Autodesk Inventor part; units mm, degrees
ref_plane "YZ Plane" through (0, 0, 0) normal (1, 0, 0) x (0, 1, 0)
ref_plane "XZ Plane" through (0, 0, 0) normal (0, 1, 0) x (-1, 0, 0)
ref_plane "XY Plane" through (0, 0, 0) normal (0, 0, 1) x (1, 0, 0)
sketch "Sketch1" plane through (0, 0, 0) normal (0, 0, 1) x (1, 0, 0)
  line L0 (0, 25.4) -> (-28.702, 25.4) construction
  line L1 (0, 25.4) -> (-86.36, 25.4) construction
  line L2 (-86.36, 25.4) -> (-80.01, 25.4) construction
  line L3 (-80.01, 25.4) -> (-73.66, 22.4389) construction
  line L4 (-80.01, 25.4) -> (-80.01, 22.4389) construction
  line L5 (-80.01, 0) -> (-86.36, 0)
  line L6 (-28.702, 59.6457) -> (-28.702, -91.9304) construction
  arc A0 (-28.9184, -4.2142) -> (-32.3684, 3.1843) centre (-35.052, -2.5707) ccw
  line L7 (-67.31, -147.4937) -> (-28.9184, -4.2142)
  line L8 (-80.01, 22.4389) -> (-73.66, 22.4389)
  line L9 (-80.01, 22.4389) -> (-80.01, 0)
  line L10 (-73.66, 22.4389) -> (-32.3684, 3.1843)
  line L11 (-28.702, -2.5707) -> (-60.452, -2.5707) construction
  line L12 (-60.452, 16.28) -> (-60.452, -121.8993) construction
  line L13 (-60.452, -121.8993) -> (-54.102, -121.8993) construction
  line L14 (-54.102, -121.8993) -> (-54.102, -98.2008) construction
  line L15 (-54.102, -98.2008) -> (-60.452, -98.2008)
  line L16 (-60.452, 16.28) -> (-60.452, 6.755) construction
  line L17 (-60.452, 16.28) -> (-60.452, 9.93) construction
  line L18 (-60.452, 9.93) -> (-46.8344, 9.93)
  line L19 (-60.452, 9.93) -> (-60.452, -98.2008)
  line L20 (-86.36, 0) -> (-86.36, -12.7) construction
  line L21 (-60.452, -12.7) -> (-73.152, -12.7) construction
  line L22 (-86.36, -12.7) -> (-86.36, -25.4) construction
  line L23 (-86.36, -25.4) -> (-86.36, -88.9) construction
  line L24 (-86.36, -88.9) -> (-73.66, -88.9) construction
  line L25 (-73.66, -88.9) -> (-73.66, -25.4) construction
  line L26 (-86.36, -25.4) -> (-73.66, -25.4)
  line L27 (-73.66, -25.4) -> (-73.66, -88.9)
  line L28 (-73.66, -88.9) -> (-86.36, -88.9)
  line L29 (-86.36, -12.7) -> (-73.152, -12.7)
  line L30 (-73.152, -133.7486) -> (-63.627, -133.7486)
  line L31 (-73.66, -88.9) -> (-73.66, -147.4937)
  line L32 (-73.66, -147.4937) -> (-67.31, -147.4937)
  line L33 (-73.152, -12.7) -> (-73.152, -133.7486)
  line L34 (-80.01, -25.4) -> (-80.01, -31.3436)
  line L35 (-80.01, -31.3436) -> (-86.36, -31.3436)
  line L36 (-86.36, 0) -> (-86.36, -25.4)
  line L37 (-86.36, -31.3436) -> (-86.36, -88.9)
  line L38 (0, -319.0244) -> (0, 122.7573)
  point P0 (0, 0)
  point P1 (-86.36, -255.9127)
  point P2 (-76.835, 22.4389)
  dimension "d0" = 28.702
  dimension "d1" = 86.36
  dimension "d2" = 6.35
  dimension "d3" = 25
  dimension "d5" = 25.4
  dimension "d6" = 25.4
  dimension "d8" = 12.7
  dimension "d11" = 6.35
  dimension "d12" = 31.75
  dimension "d13" = 6.35
  dimension "d15" = 6.35
  dimension "d16" = 12.7
  dimension "d17" = 12.7
  dimension "d18" = 12.7
  dimension "d19" = 63.5
  dimension "d20" = 12.7
  dimension "d22" = 9.525
  dimension "d23" = 6.35
  dimension "d25" = 5.9436
  dimension "d26" = 15
  dimension "d30" = 67.31
revolve "Revolution3" add sketch "Sketch1" angle 360 about axis through (0, -10, 0) along (0, 1, 0) contours L29 L33 L30 L7 L32 L31 L27 L26 L36
properties part number "Carrier Master Sketch"
For this review, take the finished solid that the model builds, in its own axes (mm). A direction names the side the tool comes from. Give positions to 0.01 mm unless a question says otherwise; leave off trailing zeros. Loops run counter-clockwise (first coordinate to the right, second up) from the corner with the lowest first, then second, coordinate; pieces in that order, holes last. Notation, with made-up numbers: M 58.25,76 L 96.25,76 A23 ccw 96.25,112 Z; hole C 21.5,46.25 d11. An arc over 180 degrees is marked long. Put each result on its own line as item: value. Start each with the question number.
(1) Wall thickness on L1, parallel to Z at x = 0, y = -69; L2, parallel to X at y = -95.5, z = 46; L3, parallel to X at y = -94, z = 3: over which ranges is each line inside the solid? List them lowest first.
(2) Add section C-C, the plane y = -48.5. Write out the cut boundary in (x, z).
(3) Machinability: for faces 1 (the cylindrical face through (15.86, -74.07, 71.41)), 2 (the flat face through (-64, -25.4, 39)), 3 (the flat face through (-32, -147.494, -60)), which of the approach directions +Z, -Z, +X, -X, +Y, -Y give a long, thin tool a straight path to every point of the face, cutting with its end or side? Answer none if there is none.
(4) Add section A-A, the plane x = 0. Write out the cut boundary in (y, z), then the cut area to 3 significant figures.
(5) For pin 1 (8 mm diameter, centred on y = -131, z = -49, fed in from +X); pin 2 (6 mm diameter, centred on x = 16, y = -97.5, fed in from +Z); pin 3 (2 mm diameter, centred on y = -51.5, z = -24, fed in from -X), all flat-tipped, find the tip position at first contact; note any pin that passes through.
(6) Add section B-B, the plane z = 0. Write out the cut boundary in (x, y), then the cut area to 3 significant figures.
Result:
1. L1: z = -73.66 to -73.15, 73.15 to 73.66
1. L2: x = -57.53 to -56.88, 56.88 to 57.53
1. L3: x = -73.6 to -73.09, 73.09 to 73.6
2. outline: C 0,0 d147.32; hole C 0,0 d146.3
3. face 1: +Y
3. face 2: -Y
3. face 3: +Z, -Z, +X, -X, -Y
4. outline: M -147.49,-73.66 L -25.4,-73.66 L -25.4,-86.36 L -12.7,-86.36 L -12.7,-73.15 L -133.75,-73.15 L -133.75,-63.63 L -147.49,-67.31 Z; M -147.49,67.31 L -133.75,63.63 L -133.75,73.15 L -12.7,73.15 L -12.7,86.36 L -25.4,86.36 L -25.4,73.66 L -147.49,73.66 Z
4. area: 671 mm^2
5. pin 1: stops at x = 58.32
5. pin 2: stops at z = 72.5
5. pin 3: stops at x = -69.98
6. outline: M -86.36,-25.4 L -73.66,-25.4 L -73.66,-147.49 L -67.31,-147.49 L -63.63,-133.75 L -73.15,-133.75 L -73.15,-12.7 L -86.36,-12.7 Z; M 63.63,-133.75 L 67.31,-147.49 L 73.66,-147.49 L 73.66,-25.4 L 86.36,-25.4 L 86.36,-12.7 L 73.15,-12.7 L 73.15,-133.75 Z
6. area: 671 mm^2
